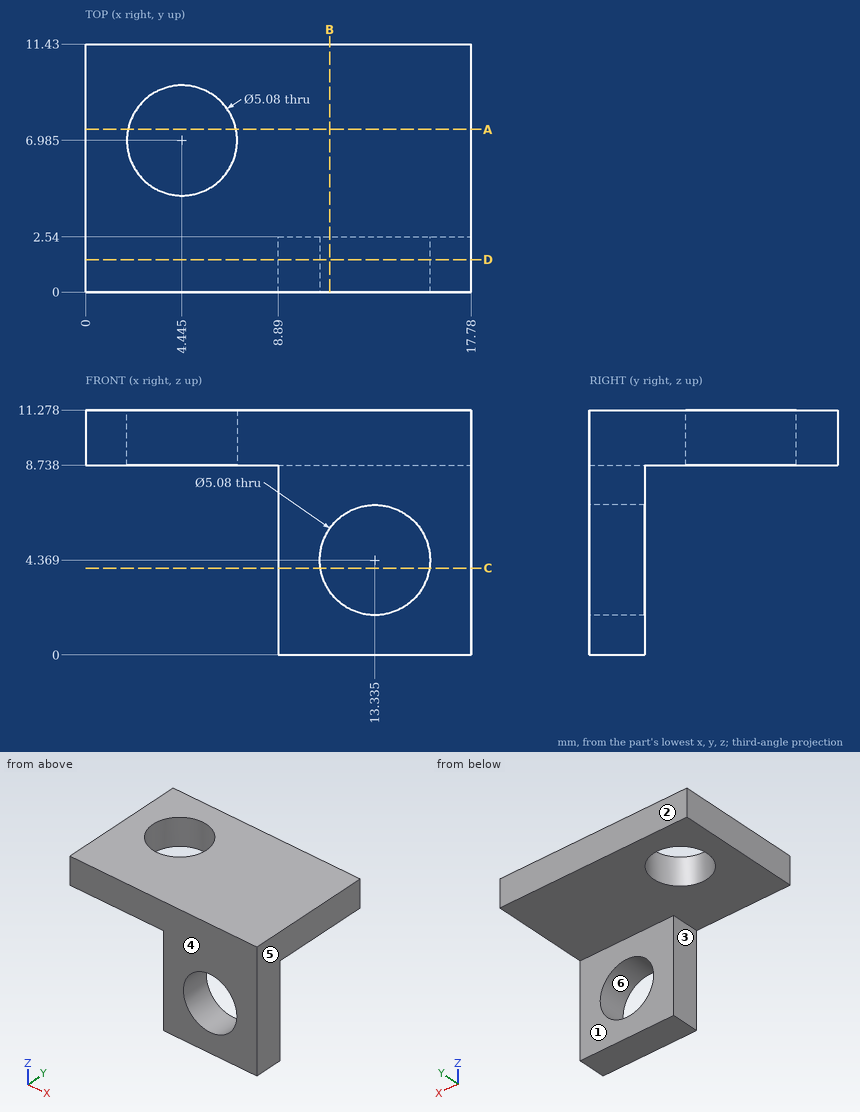
The figure shows three views and two pictorial views of one solid part (mm, origin at its lowest corner). Answer the questions. A direction names the side the tool comes from. Coordinates: 2 decimals unless noted, no trailing zeros. Loops run counter-clockwise (first coordinate to the right, second up) from the corner with the lowest first, then second, coordinate; pieces in that order, holes last. Notation, with made-up numbers: (34.5, 63) -> (41.5, 63) arc R27 ccw to (41.5, 82) -> close; hole circle Ø10 at (-20, -14.5). An arc over 180 degrees is marked (long way). Return JSON: item names as keys, results as strings. Group by question number.
(1) A cutting plane is placed at A-A on y = 7.5. Write down the section's boundary in (x, z).
(2) Which of the six approach directions +Z, -Z, +X, -X, +Y, -Y give full straight-line access (tool end or side, diameter ignored) to the marked faces 1, 2 and 3?
(3) A cutting plane is placed at C-C on z = 4. Write down the section's boundary in (x, y).
(4) A cutting plane is placed at B-B on x = 11.25. Write down the section's boundary in (y, z).
(5) Determine the mould class of the marked faces 4, 5 and 6 for opening direction X: released by +X, released by -X, zero draft, split by the parting line, or undercut.
(6) Find the intervals of material crossed by probe 1 along Z at (x, y) = (10.25, 10.25); probe 2 along Y at (x, z) = (3, 9.75) (1 decimal); probe 3 along X at (y, z) = (2, 8.5), in increasing order. Write a range as from..to.
(7) Given pin 1 Ø2.5 at (x, z) = (12, 3.5) entering from +Y; pin 2 Ø1.3 at (y, z) = (1, 6.5) entering from -X; pin 3 Ø2 at (x, z) = (6.5, 3) entering from -Y; pin 4 Ø6.5 at (x, y) = (4.445, 6.985) entering from +Z, each flat-ended and moving along its own axis, determine where each tip first touches the part or whether it passes through.
(8) A cutting plane is placed at D-D on y = 1.5. Write down the section's boundary in (x, z) (1 decimal), and give its area (3 significant figures).
The answers:
{
 "1": {"outline": "(0, 8.74) -> (1.96, 8.74) -> (1.96, 11.28) -> (0, 11.28) -> close; (6.93, 8.74) -> (17.78, 8.74) -> (17.78, 11.28) -> (6.93, 11.28) -> close"},
 "2": {"face 1": "-Z, +X, -X, +Y", "face 2": "+Z, -Z, +X, -X, +Y", "face 3": "-Z, -X, +Y, -Y"},
 "3": {"outline": "(8.89, 0) -> (10.82, 0) -> (10.82, 2.54) -> (8.89, 2.54) -> close; (15.85, 0) -> (17.78, 0) -> (17.78, 2.54) -> (15.85, 2.54) -> close"},
 "4": {"outline": "(0, 0) -> (2.54, 0) -> (2.54, 2.92) -> (0, 2.92) -> close; (0, 5.82) -> (2.54, 5.82) -> (2.54, 8.74) -> (11.43, 8.74) -> (11.43, 11.28) -> (0, 11.28) -> close"},
 "5": {"face 4": "zero draft", "face 5": "released by +X", "face 6": "undercut"},
 "6": {"probe 1": "z = 8.74..11.28", "probe 2": "y = 0..4.9, 9.1..11.4", "probe 3": "x = 8.89..17.78"},
 "7": {"pin 1": "stops at y = 2.54", "pin 2": "stops at x = 8.89", "pin 3": "passes through", "pin 4": "stops at z = 11.28"},
 "8": {"outline": "(0, 8.7) -> (8.9, 8.7) -> (8.9, 0) -> (17.8, 0) -> (17.8, 11.3) -> (0, 11.3) -> close; hole circle Ø5.1 at (13.3, 4.4)", "area": "103 mm^2"}
}
